```python
from build123d import *

# Parameters (mm, degrees)
EXTRUDE_1_DEPTH            = 4.75
EXTRUDE_START              = -4.75
SKETCH_2_W                 = 5.5
SKETCH_2_H                 = 5.5
SKETCH_2_H_2               = 8
SKETCH_2_W_2               = 8
EXTRUDE_2_DEPTH            = 9.5
EXTRUDE_3_DEPTH            = 1
HOLE_WIZARD_M61_AT_2_COUNT = 2
HOLE_WIZARD_M61_AT_2_PITCH = 18


with BuildPart() as part:
    # Эскиз1 → Бобышка-Вытянуть1 (new body, symmetric)
    with BuildSketch(Plane.XY):
        with BuildLine():
            Line((0, 50), (0, 0))
            Line((0, 0), (50, 0))
            ThreePointArc((50, 0), (48.389087297, 3.889087297), (44.5, 5.5))
            Line((44.5, 5.5), (5.5, 5.5))
            Line((5.5, 5.5), (5.5, 44.5))
            ThreePointArc((5.5, 44.5), (3.889087297, 48.389087297), (0, 50))
        make_face()
        with BuildLine():
            Line((1, 48.887482194), (1, 1))
            Line((1, 1), (48.887482194, 1))
            ThreePointArc((48.887482194, 1), (47.30624304, 3.51781182), (44.5, 4.5))
            Line((44.5, 4.5), (4.5, 4.5))
            Line((4.5, 4.5), (4.5, 44.5))
            ThreePointArc((4.5, 44.5), (3.51781182, 47.30624304), (1, 48.887482194))
        make_face(mode=Mode.SUBTRACT)
    extrude(amount=EXTRUDE_1_DEPTH, both=True)

    # Эскиз2 → Бобышка-Вытянуть2 (add)
    with BuildSketch(Plane.XY.offset(EXTRUDE_START)):
        with Locations((2.75, 2.75)):
            Rectangle(SKETCH_2_W, SKETCH_2_H)
        with Locations((2.75, 35)):
            Rectangle(SKETCH_2_W, SKETCH_2_H_2)
        with Locations((2.75, 17)):
            Rectangle(SKETCH_2_W, SKETCH_2_H_2)
        with Locations((17, 2.75)):
            Rectangle(SKETCH_2_W_2, SKETCH_2_H)
        with Locations((35, 2.75)):
            Rectangle(SKETCH_2_W_2, SKETCH_2_H)
    extrude(amount=EXTRUDE_2_DEPTH)

    # Эскиз3 → Бобышка-Вытянуть3 (add, symmetric)
    with BuildSketch(Plane.XY):
        with BuildLine():
            Line((0, 0), (50, 0))
            ThreePointArc((50, 0), (48.389087297, 3.889087297), (44.5, 5.5))
            Line((44.5, 5.5), (5.5, 5.5))
            Line((5.5, 5.5), (5.5, 44.5))
            ThreePointArc((5.5, 44.5), (3.889087297, 48.389087297), (0, 50))
            Line((0, 50), (0, 0))
        make_face()
    extrude(amount=EXTRUDE_3_DEPTH, both=True)

    # Эскиз5 → Отверстие обработанное метчиком M61 (revolve, cut)
    with BuildSketch(Plane.ZX.offset(35)):
        Polygon((0, 0), (0, 5.5), (3.1, 5.5), (2.5, 4.9), (2.5, 0.6), (3.1, 0), align=None)
    hole_wizard_m61 = revolve(axis=Axis((-6.35, 35, 0), (1, 0, 0)), mode=Mode.SUBTRACT)

    # Отверстие обработанное метчиком M61 at 2: Отверстие обработанное метчиком M61 ×2
    with Locations(*[(0, -i * HOLE_WIZARD_M61_AT_2_PITCH, 0) for i in range(1, HOLE_WIZARD_M61_AT_2_COUNT)]):
        add(hole_wizard_m61, mode=Mode.SUBTRACT)

    # Зеркальное отражение1: Отверстие обработанное метчиком M61 across plane
    add(hole_wizard_m61.mirror(Plane(origin=(0, 0, 0), x_dir=(0, 0, 1), z_dir=(-0.707106781, 0.707106781, 0))), mode=Mode.SUBTRACT)

    # Зеркальное отражение1 copy 1 sketch → Зеркальное отражение1 copy 1 (revolve, cut)
    with BuildSketch(Plane(origin=(17, 0, 0), x_dir=(0, 0, 1), z_dir=(1, 0, 0))):
        Polygon((0, 0), (0, -5.5), (3.1, -5.5), (2.5, -4.9), (2.5, -0.6), (3.1, 0), align=None)
    revolve(axis=Axis((17, -6.35, 0), (0, -1, 0)), mode=Mode.SUBTRACT)


solid = part.part
```
The listing builds one solid part. Answer for the finished solid, in the listing's coordinates (mm). A direction names the side the tool comes from. Give positions to 0.01 mm unless a question says otherwise; leave off trailing zeros. Write each loop counter-clockwise with the first axis right and the second up, starting at its lowest first coordinate (ties: lowest second). Pieces come first, ordered by that corner, then holes. Notation, with made-up numbers: (1, 8.25) - (5, 8.25) arc R15 ccw to (5, 37.25) - close; hole circle Ø1 at (-28, -20). An arc over 180 degrees is marked (long way). Use one line per item in the form item = value. Start each with the question number.
1) The mould has two halves that part along X. Classify faces 1 (the face through (5.5, 25, 0)), 2 (the face through (44, 3, -1)), 3 (the face through (4.5, 9, -3)): pulls with the +X half, pulls with the -X half, needs draft (parallel to the pull), parting line crosses it, or undercut.
2) Consider line 1 along Y through (x, z) = (7.5, 1.5); line 2 along Z through (x, y) = (3.1, 17). Determine where each line is inside the solid, lowest interval first. Write a range as from..to.
3) Find section A-A on y = 35. Determine the outline of the cut face in (x, z).
4) Find section D-D on x = 29. Determine the outline of the cut face in (y, z), plus the area to 3 significant figures.
5) Flat-ended cylindrical pins translate along their axes: pin 1 Ø4 at (y, z) = (3.5, 3) entering from +X; pin 2 Ø1 at (x, z) = (2.5, -2.5) entering from +Y; pin 3 Ø4 at (x, z) = (45, -2.5) entering from +Y. Find the tip coordinate at first contact, or state that the pin passes through.
6) Find section C-C on z = 0. Count the separate pieces of the cut face and the enclosed holes in it, plus the area to 3 significant figures.
7) A tool of negligible diameter and unlimited length cuts with its end or side. For faces 4 (the face through (31, 3, 3)), 5 (the face through (3, 13, -3)), from which of +Z, -Z, +X, -X, +Y, -Y can it reach the whole face along a straight path? Write none if from no direction.
Geometry results:
q1.face_1 = pulls with the +X half
q1.face_2 = undercut
q1.face_3 = undercut
q2.line_1 = 0..1, 4.5..5.5
q2.line_2 = -4.75..-2.5, 2.5..4.75
q3.outline = (0, -4.75) - (5.5, -4.75) - (5.5, -3.1) - (4.9, -2.5) - (0.6, -2.5) - (0, -3.1) - close; (0, 3.1) - (0.6, 2.5) - (4.9, 2.5) - (5.5, 3.1) - (5.5, 4.75) - (0, 4.75) - close
q4.outline = (0, -4.75) - (1, -4.75) - (1, -1) - (4.5, -1) - (4.5, -4.75) - (5.5, -4.75) - (5.5, 4.75) - (4.5, 4.75) - (4.5, 1) - (1, 1) - (1, 4.75) - (0, 4.75) - close
q4.area = 26.0 mm2
q5.pin_1 = 49.79
q5.pin_2 = 49.62
q5.pin_3 = 5.5
q6.separate_pieces = 5
q6.enclosed_holes = 0
q6.area = 394 mm2
q7.face_4 = +Z
q7.face_5 = -Z
